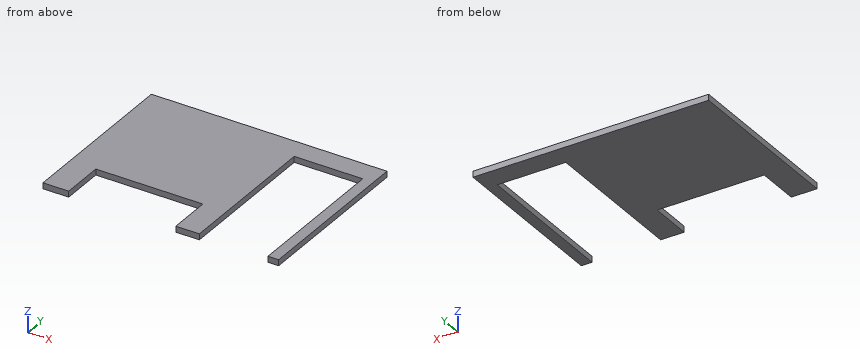
Autodesk Inventor part; units mm, degrees
ref_plane "YZ Plane" through (0, 0, 0) normal (1, 0, 0) x (0, 1, 0)
ref_plane "XZ Plane" through (0, 0, 0) normal (0, 1, 0) x (-1, 0, 0)
ref_plane "XY Plane" through (0, 0, 0) normal (0, 0, 1) x (1, 0, 0)
sketch "Sketch1" plane through (0, 0, 0) normal (0, 0, 1) x (1, 0, 0)
  line L0 (0, 0) -> (139.7, 0)
  line L1 (139.7, 0) -> (139.7, 101.6)
  line L2 (139.7, 101.6) -> (0, 101.6)
  line L3 (0, 101.6) -> (0, 0)
  dimension "d0" = 139.7
  dimension "d1" = 101.6
extrude "Extrusion1" add sketch "Sketch1" along normal blind 3.5
sketch "Sketch2" plane through (0, 0, 3.5) normal (0, 0, 1) x (1, 0, 0)
  line L0 (0, 0) -> (139.7, 0)
  line L1 (92.71, 0) -> (133.35, 0)
  line L2 (133.35, 0) -> (133.35, 88.9)
  line L3 (133.35, 88.9) -> (92.71, 88.9)
  line L4 (92.71, 88.9) -> (92.71, 0)
  line L5 (139.7, 0) -> (139.7, 101.6)
  dimension "d4" = 88.9
  dimension "d5" = 6.35
  dimension "d6" = 40.64
extrude "Extrusion2" cut sketch "Sketch2" against normal blind 3.5
sketch "Sketch3" plane through (0, 0, 3.5) normal (0, 0, 1) x (1, 0, 0)
  line L0 (15.24, 0) -> (78.74, 0)
  line L1 (78.74, 0) -> (78.74, 25.4)
  line L2 (78.74, 25.4) -> (15.24, 25.4)
  line L3 (15.24, 25.4) -> (15.24, 0)
  line L4 (133.35, 88.9) -> (133.35, 0)
  line L5 (133.35, 0) -> (139.7, 0)
  line L6 (139.7, 0) -> (139.7, 101.6)
  line L7 (139.7, 101.6) -> (0, 101.6)
  line L8 (0, 101.6) -> (0, 0)
  line L9 (0, 0) -> (92.71, 0)
  line L10 (92.71, 0) -> (92.71, 88.9)
  line L11 (92.71, 88.9) -> (133.35, 88.9)
  dimension "d9" = 25.4
  dimension "d10" = 13.97
  dimension "d11" = 63.5
  dimension "d12" = 0
extrude "Extrusion3" cut sketch "Sketch3" against normal blind 3.5 contours L3 L2 L1 L0
properties part number "CANIMDWall"
For this review, take the finished solid that the model builds, in its own axes (mm). Round coordinates to 2 decimals unless told otherwise and drop trailing zeros. Loops run counter-clockwise (first coordinate to the right, second up) from the corner with the lowest first, then second, coordinate; pieces in that order, holes last. Notation, with made-up numbers: (85.5, -19.75) - (105.5, -19.75) arc R30 cw to (105.5, 3.25) - close; hole circle Ø6 at (84, 0). An arc over 180 degrees is marked (long way). Put each result on its own line as item: value. Start each with the question number.
1. Consider section D-D on x = 23. State the section outline as (y, z) points, plus the area to 3 significant figures.
2. Consider section A-A on y = 19. State the section outline as (x, z) points.
3. Consider section B-B on y = 67.5. State the section outline as (x, z) points.
4. Consider section C-C on z = 1.4. State the section outline as (x, y) points, plus the area to 3 significant figures.
5. For probe 1 along X at (y, z) = (13.5, 2.2); probe 2 along X at (y, z) = (82.5, 2); probe 3 along Y at (x, z) = (23.5, 3.15), list the stretches that pass through material, from the lowest coordinate up. Write a range as [from, to].
Result sheet:
1. outline: (25.4, 0) - (101.6, 0) - (101.6, 3.5) - (25.4, 3.5) - close
1. area: 267 mm^2
2. outline: (0, 0) - (15.24, 0) - (15.24, 3.5) - (0, 3.5) - close; (78.74, 0) - (92.71, 0) - (92.71, 3.5) - (78.74, 3.5) - close; (133.35, 0) - (139.7, 0) - (139.7, 3.5) - (133.35, 3.5) - close
3. outline: (0, 0) - (92.71, 0) - (92.71, 3.5) - (0, 3.5) - close; (133.35, 0) - (139.7, 0) - (139.7, 3.5) - (133.35, 3.5) - close
4. outline: (0, 0) - (15.24, 0) - (15.24, 25.4) - (78.74, 25.4) - (78.74, 0) - (92.71, 0) - (92.71, 88.9) - (133.35, 88.9) - (133.35, 0) - (139.7, 0) - (139.7, 101.6) - (0, 101.6) - close
4. area: 8,970 mm^2
5. probe 1: [0, 15.24], [78.74, 92.71], [133.35, 139.7]
5. probe 2: [0, 92.71], [133.35, 139.7]
5. probe 3: [25.4, 101.6]
